For this review, take the finished solid that the model builds, in its own axes (mm). A direction names the side the tool comes from. Give positions to 0.01 mm unless a question says otherwise; leave off trailing zeros. Loops run counter-clockwise (first coordinate to the right, second up) from the corner with the lowest first, then second, coordinate; pieces in that order, holes last.
```python
from build123d import *

# Parameters (mm, degrees)
BOSS_EXTRUDE1_DEPTH = 2
SKETCH2_W           = 7
SKETCH2_H           = 3.2
BOSS_EXTRUDE2_DEPTH = 3
SKETCH3_W           = 7
SKETCH3_H           = 3.108863517
BOSS_EXTRUDE3_DEPTH = 2


with BuildPart() as part:
    # Sketch1 → Boss-Extrude1 (new body)
    with BuildSketch(Plane(origin=(0, 0, 0), x_dir=(1, 0, 0), z_dir=(0, 1, 0))):
        Polygon((-7.5, -4.5), (7.5, -4.5), (7.5, 4.5), (-7.5, 4.5), (-7.5, 5.5), (-14.5, 5.5), (-14.5, -5.5), (-7.5, -5.5), align=None)
    extrude(amount=BOSS_EXTRUDE1_DEPTH)

    # Sketch2 → Boss-Extrude2 (add)
    with BuildSketch(Plane(origin=(0, 0, 0), x_dir=(1, 0, 0), z_dir=(0, 1, 0))):
        Polygon((7.5, 4.5), (-7.5, 4.5), (-7.5, 5.5), (-14.5, 5.5), (-14.5, 3.5), (0.5, 3.5), (0.5, 3), (7.5, 3), align=None)
        Polygon((7.5, -4.5), (-7.5, -4.5), (-7.5, -5.5), (-14.5, -5.5), (-14.5, -3.5), (0.5, -3.5), (0.5, -3), (7.5, -3), align=None)
        with Locations((4, 0)):
            Rectangle(SKETCH2_W, SKETCH2_H)
    extrude(amount=-BOSS_EXTRUDE2_DEPTH)

    # Sketch3 → Boss-Extrude3 (add)
    with BuildSketch(Plane.XZ.offset(3)):
        with Locations((-11, 3.945568242)):
            Rectangle(SKETCH3_W, SKETCH3_H)
        with Locations((-11, -3.945568242)):
            Rectangle(SKETCH3_W, SKETCH3_H)
    extrude(amount=-BOSS_EXTRUDE3_DEPTH)


solid = part.part
```
Q1. For probe 1 along Z at (x, y) = (6.75, -2.4); probe 2 along Z at (x, y) = (0, -2.3); probe 3 along Y at (x, z) = (-11, 2.75), list the stretches that pass through material, from the lowest coordinate up.
Answers:
probe 1: z = -4.5 to -3, -1.6 to 1.6, 3 to 4.5
probe 2: z = -4.5 to -3.5, 3.5 to 4.5
probe 3: y = -3 to -1, 0 to 2
Q2. Mouldability with a two-part tool opening along Y and no side actions: class faces 4 (the flat face through (-11, -1, 5.5)), 5 (the flat face through (-11, -1, -3)), 6 (the flat face through (4, -3, 0)), 7 (the flat face through (-11, -1, 3)) as +Y half, -Y half, draft (parallel to the pull), parting line (faces both ways), or undercut.
Answers:
face 4: draft
face 5: undercut
face 6: -Y half
face 7: undercut
Q3. Consider section B-B on z = 1. Give the boundary of the cut face in (x, y).
Answers:
outline: (-14.5, 0) - (0.5, 0) - (0.5, -3) - (7.5, -3) - (7.5, 2) - (-14.5, 2) - close
Q4. Consider section A-A on y = -1.9. Give the boundary of the cut face in (x, z), plus the area to 3 significant figures.
Answers:
outline: (-14.5, -5.5) - (-7.5, -5.5) - (-7.5, -4.5) - (7.5, -4.5) - (7.5, -3) - (0.5, -3) - (0.5, -3.5) - (-7.5, -3.5) - (-7.5, -2.39) - (-14.5, -2.39) - close; (-14.5, 2.39) - (-7.5, 2.39) - (-7.5, 3.5) - (0.5, 3.5) - (0.5, 3) - (7.5, 3) - (7.5, 4.5) - (-7.5, 4.5) - (-7.5, 5.5) - (-14.5, 5.5) - close; (0.5, -1.6) - (7.5, -1.6) - (7.5, 1.6) - (0.5, 1.6) - close
area: 103 mm2
Q5. Machinability: for faces 1 (the flat face through (0.5, -1, 0)), 2 (the flat face through (-7.5, -1, 5)), 3 (the flat face through (-11, -2, 2.391)), which of the approach directions +Z, -Z, +X, -X, +Y, -Y give a long, thin tool a straight path to every point of the face, cutting with its end or side? Answer none if there is none.
Answers:
face 1: -X, -Y
face 2: +Z, +X, +Y, -Y
face 3: +X, -X, -Y
Q6. Consider section D-D on y = 0.9. Give the boundary of the cut face in (x, z).
Answers:
outline: (-14.5, -5.5) - (-7.5, -5.5) - (-7.5, -4.5) - (7.5, -4.5) - (7.5, 4.5) - (-7.5, 4.5) - (-7.5, 5.5) - (-14.5, 5.5) - close
Q7. Consider section C-C on x = -1. Give the boundary of the cut face in (y, z).
Answers:
outline: (-3, -4.5) - (2, -4.5) - (2, 4.5) - (-3, 4.5) - (-3, 3.5) - (0, 3.5) - (0, -3.5) - (-3, -3.5) - close
Q8. For pin 1 Ø2.5 at (x, y) = (3.5, -1) entering from +Z; pin 2 Ø1.5 at (y, z) = (-1, 1) entering from -X; pin 3 Ø1.5 at (x, y) = (-6.5, -1) entering from -Z, all flat-tipped, find the tip position at first contact; note any pin that passes through.
Answers:
pin 1: stops at z = 4.5
pin 2: stops at x = 0.5
pin 3: stops at z = -4.5
